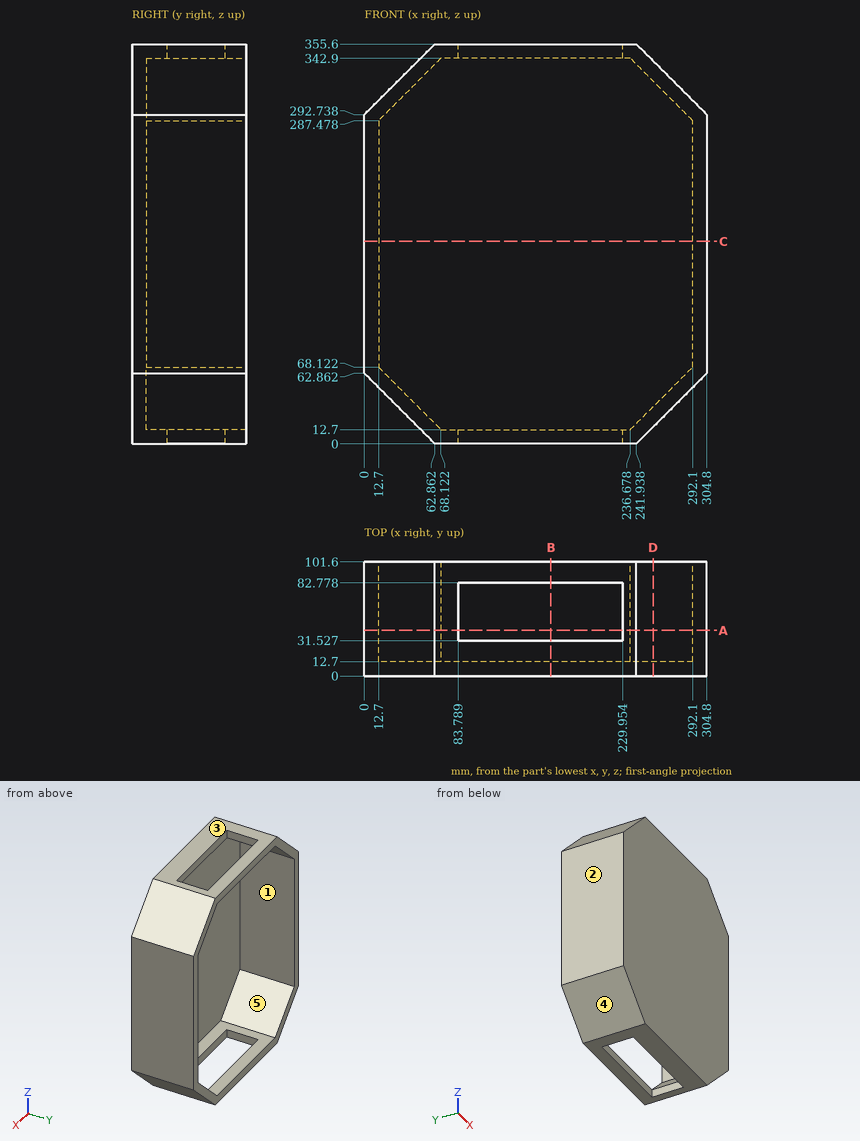
Here's the drawing with two shaded views (mm, measured from the low corner). I have some questions. A direction names the side the tool comes from. Give positions to 0.01 mm unless a question says otherwise; leave off trailing zeros. Loops run counter-clockwise (first coordinate to the right, second up) from the corner with the lowest first, then second, coordinate; pieces in that order, holes last. Notation, with made-up numbers: M 55.25,76.25 L 69.25,76.25 A3 cw 69.25,80.25 Z; hole C 83.5,-34.75 d11. An arc over 180 degrees is marked long. Answer in a Markdown table with one row per item.
1. Suppose I cut it at B-B on x = 166. Write out the boundary of the cut face in (y, z), plus the area to 3 significant figures.
Taken from the geometry:
| item | result |
|---|---|
| outline | M 0,0 L 31.53,0 L 31.53,12.7 L 12.7,12.7 L 12.7,342.9 L 31.53,342.9 L 31.53,355.6 L 0,355.6 Z; M 82.78,0 L 101.6,0 L 101.6,12.7 L 82.78,12.7 Z; M 82.78,342.9 L 101.6,342.9 L 101.6,355.6 L 82.78,355.6 Z |
| area | 5,470 mm² |
2. Which directions (+Z, -Z, +X, -X, +Y, -Y) give clear straight access to the entire face, cutting with the end or side of a thin tool? Please do the marked faces 4 and 5.
Taken from the geometry:
| item | result |
|---|---|
| face 4 | -Z, -X, +Y, -Y |
| face 5 | +Y |
3. Suppose I cut it at A-A on y = 40.5. Write out the boundary of the cut face in (x, z).
Taken from the geometry:
| item | result |
|---|---|
| outline | M 0,62.86 L 62.86,0 L 83.79,0 L 83.79,12.7 L 68.12,12.7 L 12.7,68.12 L 12.7,287.48 L 68.12,342.9 L 83.79,342.9 L 83.79,355.6 L 62.86,355.6 L 0,292.74 Z; M 229.95,0 L 241.94,0 L 304.8,62.86 L 304.8,292.74 L 241.94,355.6 L 229.95,355.6 L 229.95,342.9 L 236.68,342.9 L 292.1,287.48 L 292.1,68.12 L 236.68,12.7 L 229.95,12.7 Z |
4. Thinking about a two-plate mould opening in X: for the marked faces 1, 2 and 3, which applies, released by +X, released by -X, zero draft, split by the parting line, or undercut?
Taken from the geometry:
| item | result |
|---|---|
| face 1 | undercut |
| face 2 | released by -X |
| face 3 | zero draft |
5. For pin 1 Ø1.5 at (x, y) = (137, 31) entering from -Z; pin 2 Ø4 at (y, z) = (47, 348) entering from +X; pin 3 Ø6.5 at (y, z) = (69, 5) entering from +X; pin 4 Ø4 at (x, z) = (89.5, 157) entering from +Y, each with a flat end and sliding along its axis, tell me the tip position at first contact or that it passes through.
Taken from the geometry:
| item | result |
|---|---|
| pin 1 | stops at z = 0 |
| pin 2 | stops at x = 251.54 |
| pin 3 | stops at x = 250.19 |
| pin 4 | stops at y = 12.7 |
6. Suppose I cut it at C-C on z = 180. Write out the boundary of the cut face in (x, y).
Taken from the geometry:
| item | result |
|---|---|
| outline | M 0,0 L 304.8,0 L 304.8,101.6 L 292.1,101.6 L 292.1,12.7 L 12.7,12.7 L 12.7,101.6 L 0,101.6 Z |
7. If I drill on line 1 along X through (y, z) = (78, 82.5); line 2 along Z through (x, y) = (236.5, 28.5); line 3 along Y through (x, z) = (270.5, 183), over which ranges is the centre line in solid material (lowest first)?
Taken from the geometry:
| item | result |
|---|---|
| line 1 | x = 0 to 12.7, 292.1 to 304.8 |
| line 2 | z = 0 to 12.7, 342.9 to 355.6 |
| line 3 | y = 0 to 12.7 |
8. Suppose I cut it at D-D on x = 257. Write out the boundary of the cut face in (y, z), plus the area to 3 significant figures.
Taken from the geometry:
| item | result |
|---|---|
| outline | M 0,15.06 L 101.6,15.06 L 101.6,33.02 L 12.7,33.02 L 12.7,322.58 L 101.6,322.58 L 101.6,340.54 L 0,340.54 Z |
| area | 7,330 mm² |
